Read the model definition and answer for the solid it produces. Units are mm, in the model's axes. Face numbers are marked on the shaded views. A direction names the side the tool comes from. Coordinates: 2 decimals unless noted, no trailing zeros. Write each loop counter-clockwise with the first axis right and the second up, starting at its lowest first coordinate (ties: lowest second). Pieces come first, ordered by that corner, then holes.
Item 1: Section A-A (y = 12.5) is taken. Give the vertices of the cut face in (x, z).
Item 2: A tool of negligible diameter and unlimited length cuts with its end or side. For the marked faces 4, 5, 6 and 7, from which of +Z, -Z, +X, -X, +Y, -Y can it reach the whole face along a straight path? Write none if from no direction.
Item 3: Section B-B (x = 3.5) is taken. Give the vertices of the cut face in (y, z).
Item 4: Section C-C (z = -11) is taken. Give the vertices of the cut face in (x, y).
Item 5: Each of these flat-tipped pins is pushed along its axis until it touches: P1, Ø6, axis at y = 24, z = -12.5, coming from the +X side; P2, Ø6, axis at x = 11, z = -12.5, coming from the +Y side; P3, Ø16.5, axis at y = 29, z = 0.5, coming from the -X side. Where does it stop, or does it pass through?
Item 6: Section D-D (x = -10.5) is taken. Give the vertices of the cut face in (y, z), then the cut area to 3 significant figures.
Item 7: Straight lines are drawn through the part: probe 1 along Y at (x, z) = (-11.25, 9); probe 2 along Y at (x, z) = (3.5, 0.3); probe 3 along X at (y, z) = (5.5, 0.85). For each, find the intervals that lie inside material, in ascending order.
Item 8: Determine the mould class of the marked faces 1, 2 and 3 for opening direction X: released by +X, released by -X, zero draft, split by the parting line, or undercut.
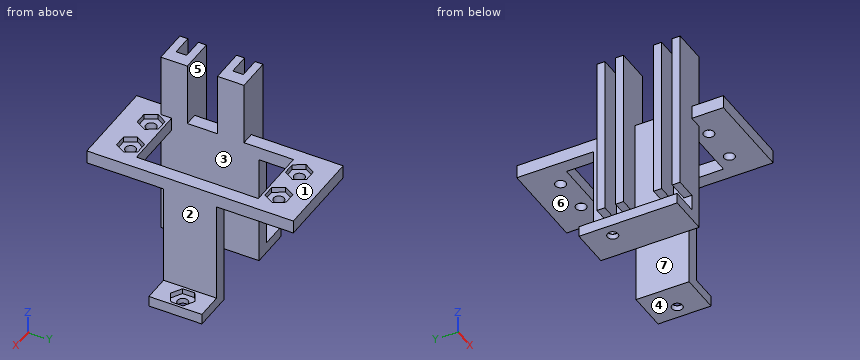
from build123d import *

# Parameters (mm, degrees)
SKETCH1_W                     = 17
SKETCH1_H                     = 39
SKETCH1_R                     = 1
SKETCH1_W_2                   = 12
SKETCH1_H_2                   = 23
SERVOBRACKET_DEPTH            = 2.5
SKETCH1_5_W                   = 2.5
SKETCH1_5_H                   = 10
SUPPORTLEGS_DEPTH             = 21.1
SKETCH2_W                     = 2
SKETCH2_H                     = 10
SUPPORTFOOT_DEPTH             = 5
SKETCH3_R                     = 1
BASEBOLTHOLE_DEPTH            = 47.581219392
SERVONUTSLOTS_DEPTH           = 1
BASENUTSLOTS_DEPTH            = 1
SKETCH6_W                     = 2.5
SKETCH6_H                     = 5
TUBEHOLDERBASE_DEPTH          = 12
SKETCH7_W                     = 4
SKETCH7_H                     = 1.5
TUBEHOLDERSTIFFENERRIBS_DEPTH = 30.6
SKETCH8_W                     = 1.5
SKETCH8_H                     = 1.5
SKETCH8_W_2                   = 1
SKETCH8_H_2                   = 1
TUBECLIPENTRANCES_DEPTH       = 1.7
SKETCH9_W                     = 0.9
SKETCH9_H                     = 1.5
TUBECLIPLOCKSLOT_DEPTH        = 0.6
SKETCH10_W                    = 0.9
SKETCH10_H                    = 1.5
TUBECLIPLOCKSLOT2_DEPTH       = 0.6
SUPPORTLEGEXTENSION_DEPTH     = 8.55


with BuildPart() as part:
    # Sketch1 → ServoBracket (new body)
    with BuildSketch(Plane.XY):
        with Locations((0, 19.5)):
            Rectangle(SKETCH1_W, SKETCH1_H)
        with Locations((-3.5, 33.5)):
            Circle(SKETCH1_R, mode=Mode.SUBTRACT)
        with Locations((-3.5, 5.5)):
            Circle(SKETCH1_R, mode=Mode.SUBTRACT)
        with Locations((3.5, 5.5)):
            Circle(SKETCH1_R, mode=Mode.SUBTRACT)
        with Locations((3.5, 33.5)):
            Circle(SKETCH1_R, mode=Mode.SUBTRACT)
        with Locations((0, 19.5)):
            Rectangle(SKETCH1_W_2, SKETCH1_H_2, mode=Mode.SUBTRACT)
    extrude(amount=SERVOBRACKET_DEPTH)

    # Sketch1<5> → SupportLegs (add)
    with BuildSketch(Plane.XY):
        with Locations((-7.25, 19.5)):
            Rectangle(SKETCH1_5_W, SKETCH1_5_H)
        with Locations((7.25, 19.5)):
            Rectangle(SKETCH1_5_W, SKETCH1_5_H)
    extrude(amount=-SUPPORTLEGS_DEPTH)

    # Sketch2 → SupportFoot (add)
    with BuildSketch(Plane.ZY.offset(8.5)):
        with Locations((-20.1, 19.5)):
            Rectangle(SKETCH2_W, SKETCH2_H)
    supportfoot = extrude(amount=SUPPORTFOOT_DEPTH)

    # Sketch3 → BaseBoltHole (cut, symmetric)
    with BuildSketch(Plane.XY.offset(-19.1)):
        with Locations((-11, 19.5)):
            Circle(SKETCH3_R)
    basebolthole = extrude(amount=BASEBOLTHOLE_DEPTH, both=True, mode=Mode.SUBTRACT)

    # SupportFoot2: SupportFoot, BaseBoltHole across plane
    add(supportfoot.mirror(Plane(origin=(0, 0, 0), x_dir=(0, 0, 1), z_dir=(1, 0, 0))))
    add(basebolthole.mirror(Plane(origin=(0, 0, 0), x_dir=(0, 0, 1), z_dir=(1, 0, 0))), mode=Mode.SUBTRACT)

    # Sketch4 → ServoNutSlots (cut)
    with BuildSketch(Plane.XY.offset(2.5)):
        Polygon((-4.654700538, 7.5), (-2.345299462, 7.5), (-1.190598923, 5.5), (-2.345299462, 3.5), (-4.654700538, 3.5), (-5.809401077, 5.5), align=None)
        Polygon((-1.190598923, 33.5), (-2.345299462, 35.5), (-4.654700538, 35.5), (-5.809401077, 33.5), (-4.654700538, 31.5), (-2.345299462, 31.5), align=None)
        Polygon((2.345299462, 31.5), (1.190598923, 33.5), (2.345299462, 35.5), (4.654700538, 35.5), (5.809401077, 33.5), (4.654700538, 31.5), align=None)
        Polygon((4.654700538, 7.5), (2.345299462, 7.5), (1.190598923, 5.5), (2.345299462, 3.5), (4.654700538, 3.5), (5.809401077, 5.5), align=None)
    extrude(amount=-SERVONUTSLOTS_DEPTH, mode=Mode.SUBTRACT)

    # Sketch5 → BaseNutSlots (cut)
    with BuildSketch(Plane.XY.offset(-19.1)):
        Polygon((-11, 21.809401077), (-13, 20.654700538), (-13, 18.345299462), (-11, 17.190598923), (-9, 18.345299462), (-9, 20.654700538), align=None)
        Polygon((11, 21.809401077), (9, 20.654700538), (9, 18.345299462), (11, 17.190598923), (13, 18.345299462), (13, 20.654700538), align=None)
    extrude(amount=-BASENUTSLOTS_DEPTH, mode=Mode.SUBTRACT)

    # Sketch6 → TubeHolderBase (add)
    with BuildSketch(Plane.XY.offset(2.5)):
        with Locations((-7.25, 19.15)):
            Rectangle(SKETCH6_W, SKETCH6_H)
    tubeholderbase = extrude(amount=TUBEHOLDERBASE_DEPTH)

    # Sketch7 → TubeHolderStiffenerRibs (add)
    with BuildSketch(Plane.XY.offset(14.5)):
        with Locations((-10.5, 20.9)):
            Rectangle(SKETCH7_W, SKETCH7_H)
        with Locations((-10.5, 17.4)):
            Rectangle(SKETCH7_W, SKETCH7_H)
    tubeholderstiffenerribs = extrude(amount=-TUBEHOLDERSTIFFENERRIBS_DEPTH)

    # TubeHolder2: TubeHolderBase, TubeHolderStiffenerRibs across plane
    add(tubeholderbase.mirror(Plane.ZX.offset(13.8)))
    add(tubeholderstiffenerribs.mirror(Plane.ZX.offset(13.8)))

    # Sketch8 → TubeClipEntrances (cut)
    # profile 1 of 4: a face of its own
    with BuildSketch(Plane.ZY.offset(8.5)):
        with Locations((10.3, 19.15)):
            Rectangle(SKETCH8_W, SKETCH8_H)
        with Locations((10.3, 19.15)):
            Rectangle(SKETCH8_W_2, SKETCH8_H_2, mode=Mode.SUBTRACT)
    # profile 2 of 4: a face of its own
    with BuildSketch(Plane.ZY.offset(8.5)):
        with Locations((10.3, 19.15)):
            Rectangle(SKETCH8_W_2, SKETCH8_H_2)
    # profile 3 of 4: a face of its own
    with BuildSketch(Plane.ZY.offset(8.5)):
        with Locations((11.1, 8.45)):
            Rectangle(SKETCH8_W, SKETCH8_H)
        with Locations((11.1, 8.45)):
            Rectangle(SKETCH8_W_2, SKETCH8_H_2, mode=Mode.SUBTRACT)
    # profile 4 of 4: a face of its own
    with BuildSketch(Plane.ZY.offset(8.5)):
        with Locations((11.1, 8.45)):
            Rectangle(SKETCH8_W_2, SKETCH8_H_2)
    extrude(amount=-TUBECLIPENTRANCES_DEPTH, mode=Mode.SUBTRACT)

    # Sketch9 → TubeClipLockSlot (cut)
    with BuildSketch(Plane(origin=(0, 0, 11.05), x_dir=(-1, 0, 0), z_dir=(0, 0, -1))):
        with Locations((7.25, 19.15)):
            Rectangle(SKETCH9_W, SKETCH9_H)
    extrude(amount=-TUBECLIPLOCKSLOT_DEPTH, mode=Mode.SUBTRACT)

    # Sketch10 → TubeClipLockSlot2 (cut)
    with BuildSketch(Plane(origin=(0, 0, 11.85), x_dir=(-1, 0, 0), z_dir=(0, 0, -1))):
        with Locations((7.25, 8.45)):
            Rectangle(SKETCH10_W, SKETCH10_H)
    extrude(amount=-TUBECLIPLOCKSLOT2_DEPTH, mode=Mode.SUBTRACT)

    # Sketch11 → SupportLegExtension (add)
    with BuildSketch(Plane.XZ.offset(-14.5)):
        Polygon((-6, 0), (-8.5, 0), (-8.5, -19.1), (-13.5, -19.1), (-13.5, -21.1), (-6, -21.1), align=None)
    extrude(amount=SUPPORTLEGEXTENSION_DEPTH)


solid = part.part
Established:
1. outline: (-13.5, -21.1) - (-6, -21.1) - (-6, 2.5) - (-8.5, 2.5) - (-8.5, -19.1) - (-13.5, -19.1) - close; (6, 0) - (8.5, 0) - (8.5, 2.5) - (6, 2.5) - close
2. face 4: -Z, +X, -X, +Y, -Y
2. face 5: +Z, -X
2. face 6: -Z, +X, -X, +Y
2. face 7: +Z, -Z
3. outline: (0, 0) - (4.5, 0) - (4.5, 1.5) - (3.5, 1.5) - (3.5, 2.5) - (0, 2.5) - close; (6.5, 0) - (8, 0) - (8, 2.5) - (7.5, 2.5) - (7.5, 1.5) - (6.5, 1.5) - close; (31, 0) - (32.5, 0) - (32.5, 1.5) - (31.5, 1.5) - (31.5, 2.5) - (31, 2.5) - close; (34.5, 0) - (39, 0) - (39, 2.5) - (35.5, 2.5) - (35.5, 1.5) - (34.5, 1.5) - close
4. outline: (-12.5, 5.95) - (-6, 5.95) - (-6, 24.5) - (-8.5, 24.5) - (-8.5, 21.65) - (-12.5, 21.65) - (-12.5, 20.15) - (-8.5, 20.15) - (-8.5, 18.15) - (-12.5, 18.15) - (-12.5, 16.65) - (-8.5, 16.65) - (-8.5, 10.95) - (-12.5, 10.95) - (-12.5, 9.45) - (-8.5, 9.45) - (-8.5, 7.45) - (-12.5, 7.45) - close; (6, 14.5) - (8.5, 14.5) - (8.5, 24.5) - (6, 24.5) - close
5. P1: stops at x = 8.5
5. P2: stops at y = 24.5
5. P3: stops at x = -12.5
6. outline: (5.95, -21.1) - (18.63, -21.1) - (18.63, -20.1) - (17.48, -20.1) - (17.48, -19.1) - (5.95, -19.1) - close; (5.95, -16.1) - (7.45, -16.1) - (7.45, 14.5) - (5.95, 14.5) - close; (9.45, -16.1) - (10.95, -16.1) - (10.95, 14.5) - (9.45, 14.5) - close; (16.65, -16.1) - (18.15, -16.1) - (18.15, 14.5) - (16.65, 14.5) - close; (20.15, -16.1) - (21.65, -16.1) - (21.65, 14.5) - (20.15, 14.5) - close; (20.37, -21.1) - (24.5, -21.1) - (24.5, -19.1) - (21.52, -19.1) - (21.52, -20.1) - (20.37, -20.1) - close
6. area: 215 mm2
7. probe 1: y = 5.95 to 7.45, 9.45 to 10.95, 16.65 to 18.15, 20.15 to 21.65
7. probe 2: y = 0 to 4.5, 6.5 to 8, 31 to 32.5, 34.5 to 39
7. probe 3: x = -8.5 to -4.5, -2.5 to 2.5, 4.5 to 8.5
8. face 1: zero draft
8. face 2: released by +X
8. face 3: undercut
